Geometry check sheet. Reference: the model listing, model coordinates, mm. Face numbers are marked on the shaded views. Round coordinates to 2 decimals unless told otherwise and drop trailing zeros. Order: outer loops, then holes, each group sorted by start corner. A loop starts at its lowest first (then second) coordinate and runs counter-clockwise, first axis right, second up. Notation, with made-up numbers: (35.25, 71.5) -> (90.25, 71.5) arc R21 ccw to (90.25, 108.5) -> close; hole circle Ø11 at (6, 36). An arc over 180 degrees is marked (long way). Use a Markdown table: item, result. Add a question column.
Item 1: Sectioned sample at C-C, the plane z = -48. Record the cut outline in (x, y), and give its area (3 significant figures).
Item 2: Sectioned sample at A-A, the plane y = 32.5. Record the cut outline in (x, z).
Item 3: Sectioned sample at D-D, the plane x = 12. Record the cut outline in (y, z), and give its area (3 significant figures).
Item 4: Mould release check, pull along X, two halves, no side actions. Record for the marked faces 1, 2 and 3: pulls with the +X half, pulls with the -X half, needs draft (parallel to the pull), parting line crosses it, or undercut.
Item 5: Gauge pin test, flat ends, axial feed: pin 1 Ø12 at (x, z) = (26, -19.5) entering from +Y; pin 2 Ø4 at (x, z) = (25, -79) entering from -Y; pin 3 Ø2 at (x, y) = (38, 1) entering from +Z. Record the tip position at first contact, or that the pin passes through.
Item 6: Sectioned sample at B-B, the plane z = -20.5. Record the cut outline in (x, y).
Item 7: Material ranges on probe 1 along X at (y, z) = (32.5, -49); probe 2 along Y at (x, z) = (-25, -83), recorded low to high. Write a range as [from, to].
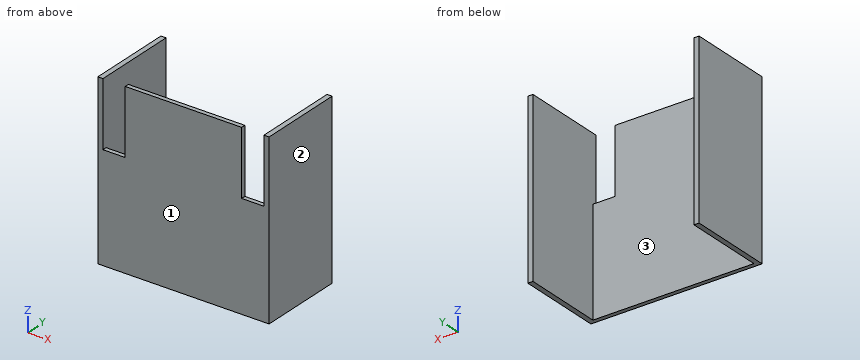
from build123d import *

# Parameters (mm, degrees)
SALIENTE_EXTRUIR1_DEPTH = 100
CROQUIS2_W              = 13
CROQUIS2_H              = 38
CORTAR_EXTRUIR2_DEPTH   = 10


with BuildPart() as part:
    # Croquis1 → Saliente-Extruir1 (new body)
    with BuildSketch(Plane.XY):
        Polygon((50, 0), (-50, 0), (-50, 50), (-47, 50), (-47, 2.5), (47, 2.5), (47, 50), (50, 50), align=None)
    extrude(amount=-SALIENTE_EXTRUIR1_DEPTH)

    # Croquis2 → Cortar-Extruir2 (cut)
    with BuildSketch(Plane(origin=(0, 2.5, 0), x_dir=(1, 0, 0), z_dir=(0, 1, 0))):
        with Locations((-40.5, 19)):
            Rectangle(CROQUIS2_W, CROQUIS2_H)
        with Locations((40.5, 19)):
            Rectangle(CROQUIS2_W, CROQUIS2_H)
    extrude(amount=-CORTAR_EXTRUIR2_DEPTH, mode=Mode.SUBTRACT)


solid = part.part
Found:
| question | item | result |
|---|---|---|
| 1 | outline | (-50, 0) -> (50, 0) -> (50, 50) -> (47, 50) -> (47, 2.5) -> (-47, 2.5) -> (-47, 50) -> (-50, 50) -> close |
| 1 | area | 535 mm2 |
| 2 | outline | (-50, -100) -> (-47, -100) -> (-47, 0) -> (-50, 0) -> close; (47, -100) -> (50, -100) -> (50, 0) -> (47, 0) -> close |
| 3 | outline | (0, -100) -> (2.5, -100) -> (2.5, 0) -> (0, 0) -> close |
| 3 | area | 250 mm2 |
| 4 | face 1 | needs draft |
| 4 | face 2 | pulls with the +X half |
| 4 | face 3 | undercut |
| 5 | pin 1 | stops at y = 2.5 |
| 5 | pin 2 | stops at y = 0 |
| 5 | pin 3 | stops at z = -38 |
| 6 | outline | (-50, 0) -> (-47, 0) -> (-47, 50) -> (-50, 50) -> close; (-34, 0) -> (34, 0) -> (34, 2.5) -> (-34, 2.5) -> close; (47, 0) -> (50, 0) -> (50, 50) -> (47, 50) -> close |
| 7 | probe 1 | x = [-50, -47], [47, 50] |
| 7 | probe 2 | y = [0, 2.5] |
